Here's the drawing with two shaded views (mm, measured from the low corner). I have some questions. A direction names the side the tool comes from. Coordinates: 2 decimals unless noted, no trailing zeros. Write each loop counter-clockwise with the first axis right and the second up, starting at its lowest first coordinate (ties: lowest second). Pieces come first, ordered by that corner, then holes.
Item 1: If we section it at C-C (y = 12.5): Please give me the cut outline in (x, z).
Item 2: For the marked faces 1, 2 and 3, which set-ups out of +Z, -Z, +X, -X, +Y, -Y let a thin tool reach every point of the face, with its end or its side?
Item 3: If we section it at B-B (z = 12.7): Please give me the cut outline in (x, y).
Item 4: We'd pull the mould along X, two halves only. Please class the marked faces 4, 5 and 6: +X half, -X half, draft (parallel to the pull), parting line (faces both ways), or undercut.
Item 5: I'm going to push flat-ended pins straight in: pin 1 Ø4 at (x, z) = (52.705, 25.4) entering from -Y; pin 2 Ø10 at (y, z) = (28, 45) entering from -X (3 decimals); pin 3 Ø6 at (x, z) = (63, 71) entering from +Y. Where does each tip first touch, or does it pass through?
Item 6: If we section it at D-D (x = 72): Please give me the cut outline in (y, z).
Item 7: If I drill on line 1 (X direction, y = 32.3, z = 12.7); line 2 (X direction, y = 26.5, z = 5); line 3 (Y direction, x = 15.5, z = 24), over which ranges is the centre line in solid material (lowest first)?
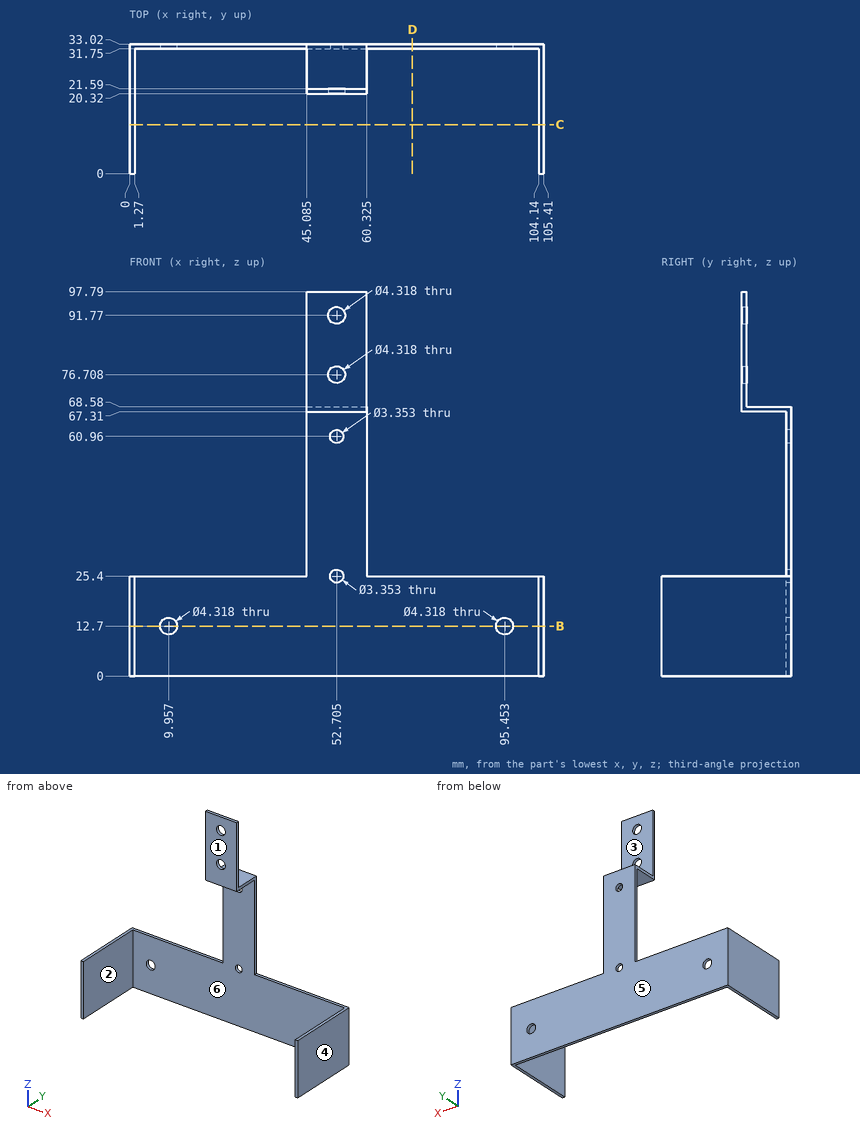
Answer list:
1. outline: (0, 0) - (1.27, 0) - (1.27, 25.4) - (0, 25.4) - close; (104.14, 0) - (105.41, 0) - (105.41, 25.4) - (104.14, 25.4) - close
2. face 1: +Z, -Z, +X, -X, -Y
2. face 2: +Z, -Z, -Y
2. face 3: +Z, +X, -X, +Y
3. outline: (0, 0) - (1.27, 0) - (1.27, 31.75) - (7.8, 31.75) - (7.8, 33.02) - (0, 33.02) - close; (12.12, 31.75) - (93.29, 31.75) - (93.29, 33.02) - (12.12, 33.02) - close; (97.61, 31.75) - (104.14, 31.75) - (104.14, 0) - (105.41, 0) - (105.41, 33.02) - (97.61, 33.02) - close
4. face 4: +X half
4. face 5: draft
4. face 6: undercut
5. pin 1: stops at y = 31.75
5. pin 2: stops at x = 45.085
5. pin 3: stops at y = 21.59
6. outline: (31.75, 0) - (33.02, 0) - (33.02, 25.4) - (31.75, 25.4) - close
7. line 1: x = 0 to 7.8, 12.12 to 93.29, 97.61 to 105.41
7. line 2: x = 0 to 1.27, 104.14 to 105.41
7. line 3: y = 31.75 to 33.02
